Work out the finished part from the listing and answer in its coordinate system (mm). A direction names the side the tool comes from. Round coordinates to 2 decimals unless told otherwise and drop trailing zeros. Order: outer loops, then holes, each group sorted by start corner. A loop starts at its lowest first (then second) coordinate and runs counter-clockwise, first axis right, second up. Notation, with made-up numbers: M 36,-36.5 L 72,-36.5 A31 ccw 72,-3.5 Z; hole C 50,73.25 d4. An arc over 180 degrees is marked long. Return JSON: item names as keys, results as strings.
from build123d import *

# Parameters (mm, degrees)
SKETCH_1_W          = 40
SKETCH_1_H          = 40
EXTRUDE_1_DEPTH     = 9
SKETCH_2_W          = 4.7
SKETCH_2_H          = 40
EXTRUDE_2_DEPTH     = 40
CUT_EXTRUDE_START   = -28.6
CUT_EXTRUDE_2_DEPTH = 28.6
SKETCH_4_R          = 4
CUT_EXTRUDE_3_DEPTH = 64.067344958
SKETCH_6_R          = 4
CUT_EXTRUDE_5_DEPTH = 49.989794856
SKETCH_7_W          = 8.2
SKETCH_7_H          = 1
EXTRUDE_3_DEPTH     = 2


# Read off the part's stored shape, not the designer's step: 切除-拉伸2
with BuildPart() as part:
    # 草图1 → 凸台-拉伸1 (new body)
    with BuildSketch(Plane.XY):
        Rectangle(SKETCH_1_W, SKETCH_1_H)
    extrude(amount=EXTRUDE_1_DEPTH)

    # 草图2 → 凸台-拉伸2 (add)
    with BuildSketch(Plane.XY.offset(9)):
        with Locations((-11.95, 0)):
            Rectangle(SKETCH_2_W, SKETCH_2_H)
        with Locations((11.95, 0)):
            Rectangle(SKETCH_2_W, SKETCH_2_H)
    extrude(amount=EXTRUDE_2_DEPTH)

    # 切除-拉伸2 outline → 切除-拉伸2 (cut)
    with BuildSketch(Plane.ZY.offset(14.3).offset(CUT_EXTRUDE_START)):
        with BuildLine():
            Line((49, 20), (29, 20))
            ThreePointArc((29, 20), (43.142135559, 14.142135688), (49, 1.83e-07))
            Line((49, 1.83e-07), (49, 20))
        make_face()
        with BuildLine():
            Line((49, -20), (49, 1.83e-07))
            ThreePointArc((49, 1.83e-07), (43.142135688, -14.142135559), (29, -20))
            Line((29, -20), (49, -20))
        make_face()
    extrude(amount=CUT_EXTRUDE_2_DEPTH, mode=Mode.SUBTRACT)

    # 草图4 → 切除-拉伸3 (cut, through all)
    with BuildSketch(Plane.ZY.offset(14.3)):
        with Locations((29, 0)):
            Circle(SKETCH_4_R)
    extrude(amount=-CUT_EXTRUDE_3_DEPTH, mode=Mode.SUBTRACT)

    # 草图6 → 切除-拉伸5 (cut, through all)
    with BuildSketch(Plane.XY.offset(9)):
        Circle(SKETCH_6_R)
    extrude(amount=-CUT_EXTRUDE_5_DEPTH, mode=Mode.SUBTRACT)

    # 草图7 → 凸台-拉伸3 (add)
    with BuildSketch(Plane(origin=(0, 0, 0), x_dir=(-1, 0, 0), z_dir=(0, 0, -1))):
        with Locations((0, 19.5)):
            Rectangle(SKETCH_7_W, SKETCH_7_H)
        with Locations((0, -19.5)):
            Rectangle(SKETCH_7_W, SKETCH_7_H)
    extrude(amount=EXTRUDE_3_DEPTH)


solid = part.part
Item 1: Find section A-A (x = 0). Determine the outline of the cut face in (y, z), plus the area to 3 significant figures.
Output:
{"outline": "M -20,-2 L -19,-2 L -19,0 L -4,0 L -4,9 L -20,9 Z; M 4,0 L 19,0 L 19,-2 L 20,-2 L 20,9 L 4,9 Z", "area": "292 mm^2"}
Item 2: Each of these flat-tipped pins is pushed along its axis until it touches: pin 1 (10 mm diameter, centred on x = 4, y = 5, fed in from -Z); pin 2 (1.1 mm diameter, centred on y = -19.5, z = -1.5, fed in from -X); pin 3 (12 mm diameter, centred on y = -9.5, z = 34.5, fed in from +X). Where does it stop, or does it pass through?
Output:
{"pin 1": "stops at z = 0", "pin 2": "stops at x = -4.1", "pin 3": "stops at x = 14.3"}
Item 3: Which of the six approach directions +Z, -Z, +X, -X, +Y, -Y give full straight-line access (tool end or side, diameter ignored) to faces 5 (the flat face through (17, 0, 9)), 6 (the flat face through (-14.3, 0, 24)), 7 (the flat face through (-4.4, 0.3, 9))?
Output:
{"face 5": "+Z, +X, +Y, -Y", "face 6": "+Z, -X, +Y, -Y", "face 7": "+Z, +Y, -Y"}
Item 4: Consider line 1 along X through (y, z) = (-16, 39); line 2 along Y through (x, z) = (0, 6.25); line 3 along Z through (x, y) = (5, 14). Determine where each line is inside the solid, lowest interval first. Write a range as [from, to].
Output:
{"line 1": "x = [-14.3, -9.6], [9.6, 14.3]", "line 2": "y = [-20, -4], [4, 20]", "line 3": "z = [0, 9]"}
Item 5: Find section D-D (z = 27). Determine the outline of the cut face in (x, y).
Output:
{"outline": "M -14.3,-20 L -9.6,-20 L -9.6,-3.46 L -14.3,-3.46 Z; M -14.3,3.46 L -9.6,3.46 L -9.6,20 L -14.3,20 Z; M 9.6,-20 L 14.3,-20 L 14.3,-3.46 L 9.6,-3.46 Z; M 9.6,3.46 L 14.3,3.46 L 14.3,20 L 9.6,20 Z"}
Item 6: Find section B-B (x = 13). Determine the outline of the cut face in (y, z), plus the area to 3 significant figures.
Output:
{"outline": "M -20,0 L 20,0 L 20,29 A20 ccw -20,29 Z; hole C 0,29 d8", "area": "1,740 mm^2"}
Item 7: Find section C-C (y = -1.5). Determine the outline of the cut face in (x, z).
Output:
{"outline": "M -20,0 L -3.71,0 L -3.71,9 L -9.6,9 L -9.6,25.29 L -14.3,25.29 L -14.3,9 L -20,9 Z; M -14.3,32.71 L -9.6,32.71 L -9.6,48.94 L -14.3,48.94 Z; M 3.71,0 L 20,0 L 20,9 L 14.3,9 L 14.3,25.29 L 9.6,25.29 L 9.6,9 L 3.71,9 Z; M 9.6,32.71 L 14.3,32.71 L 14.3,48.94 L 9.6,48.94 Z"}
Item 8: The mould has two halves that part along X. Classify faces 1 (the flat face through (-20, 0, 4)), 2 (the cylindrical face through (-0.867, -3.905, 4.563)), 3 (the flat face through (0, 19, -1)), 4 (the flat face through (9.6, 0, 24)): pulls with the +X half, pulls with the -X half, needs draft (parallel to the pull), parting line crosses it, or undercut.
Output:
{"face 1": "pulls with the -X half", "face 2": "undercut", "face 3": "needs draft", "face 4": "undercut"}
